Verification items for the finished model (mm, model axes). A direction names the side the tool comes from. Give positions to 0.01 mm unless a question says otherwise; leave off trailing zeros. Order: outer loops, then holes, each group sorted by start corner. A loop starts at its lowest first (then second) coordinate and runs counter-clockwise, first axis right, second up. Notation, with made-up numbers: (84, 13.25) - (92, 13.25) arc R21 cw to (92, 46.25) - close; hole circle Ø2 at (43, 63.5). An arc over 180 degrees is marked (long way). Answer as a JSON object with one key per item and string values. Group by question number.
(1) Depth check by flat-ended pin: pin 1 Ø4 at (x, z) = (2.5, -2.5) entering from -Y; pin 2 Ø1.5 at (y, z) = (-35.5, 2.5) entering from -X; pin 3 Ø0.7 at (x, y) = (-0.5, -2) entering from -Z. Enter the tip coordinate at first touch or a pass-through.
(2) Thickness scan on line 1 (Y direction, x = 2.25, z = 0.25); line 2 (Y direction, x = -0.5, z = 0.25); line 3 (Z direction, x = 1.5, y = -23). Record the ranges inside material, lowest first.
(3) Section check B-B (y = -29). Record the boundary of the cut face in (x, z).
(4) Section check A-A (x = 0). Record the boundary of the cut face in (y, z), then the cut area to 3 significant figures.
(5) Access from +Z, -Z, +X, -X, +Y, -Y to the whole of each face (thin tool, end or side, straight path). Record for faces 1 (the face through (0, -23, -2)), 2 (the face through (0, -3, 0)), 3 (the face through (-2, 0, -1)).
(6) Mould release check, pull along X, two halves, no side actions. Record for faces 4 (the face through (3.233, -2.276, -1.341)), 5 (the face through (0, -44, 0)), 6 (the face through (1.724, -1.479, 1.014)): +X half, -X half, draft (parallel to the pull), parting line (faces both ways), or undercut.
```python
from build123d import *

# Parameters (mm, degrees)
F0_R     = 3.5
F1_DEPTH = 4
F2_R     = 2
F3_DEPTH = 40
F5_DEPTH = 3
F6_SIZE  = 0.6


with BuildPart() as f1:
    # F0 (on Front) → F1 (new body)
    with BuildSketch(Plane.XZ):
        Circle(F0_R)
    extrude(amount=F1_DEPTH)

    # F2 (on face) → F3 (join)
    with BuildSketch(Plane.XZ.offset(4)):
        Circle(F2_R)
    extrude(amount=F3_DEPTH)

    # F4 (on face) → F5 (cut)
    with BuildSketch(Plane(origin=(0, 0, 0), x_dir=(-1, 0, 0), z_dir=(0, 1, 0))):
        Polygon((1.154701, 2), (-1.154701, 2), (-2.309401, 0), (-1.154701, -2), (1.154701, -2), (2.309401, 0), align=None)
    extrude(amount=-F5_DEPTH, mode=Mode.SUBTRACT)

    # F6
    f6_edges = [f1.edges().sort_by_distance(p)[0] for p in [
        (-3.5, 0, 0),
        (-2, -44, 0),
    ]]
    chamfer(f6_edges, length=F6_SIZE)


solid = f1.part
```
Solutions:
{
 "1": {"pin 1": "stops at y = -43.86", "pin 2": "stops at x = -0.97", "pin 3": "stops at z = -3.5"},
 "2": {"line 1": "y = -4 to 0", "line 2": "y = -44 to -3", "line 3": "z = -1.32 to 1.32"},
 "3": {"outline": "circle Ø4 at (0, 0)"},
 "4": {"outline": "(-44, -1.4) - (-43.4, -2) - (-4, -2) - (-4, -3.5) - (-0.6, -3.5) - (0, -2.9) - (0, -2) - (-3, -2) - (-3, 2) - (0, 2) - (0, 2.9) - (-0.6, 3.5) - (-4, 3.5) - (-4, 2) - (-43.4, 2) - (-44, 1.4) - close", "area": "175 mm2"},
 "5": {"face 1": "-Y", "face 2": "+Y", "face 3": "+Z, -Z, +X, -X, +Y"},
 "6": {"face 4": "parting line", "face 5": "draft", "face 6": "undercut"}
}
